Geometry check sheet. Reference: the model listing, model coordinates, mm. Face numbers are marked on the shaded views. Coordinates: 2 decimals unless noted, no trailing zeros. Write each loop counter-clockwise with the first axis right and the second up, starting at its lowest first coordinate (ties: lowest second). Pieces come first, ordered by that corner, then holes. Notation, with made-up numbers: (-34, 37) -> (-15, 37) arc R14 ccw to (-15, 51) -> close; hole circle Ø7 at (70, 18.25). An arc over 180 degrees is marked (long way). Answer as CSV lines item,"result".
```python
from build123d import *

# Parameters (mm, degrees)
SKETCH1_R           = 30.5
SKETCH1_R_2         = 17.5
BOSS_EXTRUDE1_DEPTH = 15
SKETCH2_R           = 2
CUT_EXTRUDE1_DEPTH  = 15
FILLET1_R           = 1
FILLET2_R           = 0.5


with BuildPart() as part:
    # Sketch1 → Boss-Extrude1 (new body)
    with BuildSketch(Plane(origin=(0, 0, 0), x_dir=(1, 0, 0), z_dir=(0, 1, 0))):
        with Locations(Location((0, 0, 0), (0, 0, 270))):
            Circle(SKETCH1_R)
        with Locations(Location((0, 0, 0), (0, 0, 270))):
            Circle(SKETCH1_R_2, mode=Mode.SUBTRACT)
    extrude(amount=BOSS_EXTRUDE1_DEPTH)

    # Sketch2 → Cut-Extrude1 (cut)
    with BuildSketch(Plane(origin=(0, 15, 0), x_dir=(1, 0, 0), z_dir=(0, 1, 0))):
        with Locations(Location((0, 22.5, 0), (0, 0, 270))):
            Circle(SKETCH2_R)
        with Locations(Location((15.909902577, 15.909902577, 0), (0, 0, 270))):
            Circle(SKETCH2_R)
        with Locations(Location((22.5, 0, 0), (0, 0, 270))):
            Circle(SKETCH2_R)
        with Locations(Location((15.909902577, -15.909902577, 0), (0, 0, 270))):
            Circle(SKETCH2_R)
        with Locations(Location((0, -22.5, 0), (0, 0, 270))):
            Circle(SKETCH2_R)
        with Locations(Location((-15.909902577, -15.909902577, 0), (0, 0, 270))):
            Circle(SKETCH2_R)
        with Locations(Location((-22.5, 0, 0), (0, 0, 270))):
            Circle(SKETCH2_R)
        with Locations(Location((-15.909902577, 15.909902577, 0), (0, 0, 270))):
            Circle(SKETCH2_R)
    extrude(amount=-CUT_EXTRUDE1_DEPTH, mode=Mode.SUBTRACT)

    # Fillet1
    fillet1_edges = [part.edges().sort_by_distance(p)[0] for p in [
        (0, 0, -17.5),
        (0, 15, -17.5),
    ]]
    fillet(fillet1_edges, radius=FILLET1_R)

    # Fillet2
    fillet2_edges = [part.edges().sort_by_distance(p)[0] for p in [
        (0, 0, -30.5),
        (0, 15, -30.5),
    ]]
    fillet(fillet2_edges, radius=FILLET2_R)


solid = part.part
```
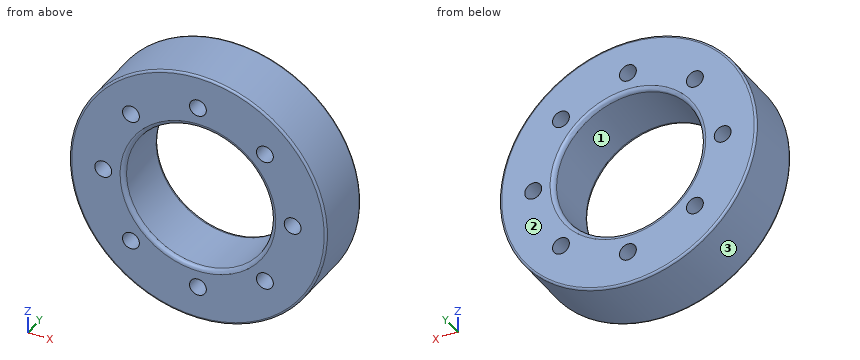
Item 1: Thickness scan on probe 1 along X at (y, z) = (10, 0); probe 2 along Z at (x, y) = (15.5, 10.5); probe 3 along Z at (x, y) = (23, 3.25). Record the ranges inside material, lowest first.
Responses:
probe 1,"x = -30.5 to -24.5, -20.5 to -17.5, 17.5 to 20.5, 24.5 to 30.5"
probe 2,"z = -26.27 to -17.87, -13.95 to -8.12, 8.12 to 13.95, 17.87 to 26.27"
probe 3,"z = -20.03 to -1.94, 1.94 to 20.03"
Item 2: Cross-section at A-A, the plane z = 0. Record the cut outline in (x, y).
Responses:
outline,"(-30.5, 0.5) arc R0.5 ccw to (-30, 0) -> (-24.5, 0) -> (-24.5, 15) -> (-30, 15) arc R0.5 ccw to (-30.5, 14.5) -> close; (-20.5, 0) -> (-18.5, 0) arc R1 ccw to (-17.5, 1) -> (-17.5, 14) arc R1 ccw to (-18.5, 15) -> (-20.5, 15) -> close; (17.5, 1) arc R1 ccw to (18.5, 0) -> (20.5, 0) -> (20.5, 15) -> (18.5, 15) arc R1 ccw to (17.5, 14) -> close; (24.5, 0) -> (30, 0) arc R0.5 ccw to (30.5, 0.5) -> (30.5, 14.5) arc R0.5 ccw to (30, 15) -> (24.5, 15) -> close"
Item 3: Depth check by flat-ended pin: pin 1 Ø4.5 at (x, z) = (15.91, 15.91) entering from +Y; pin 2 Ø5 at (y, z) = (9.5, 7) entering from -X; pin 3 Ø1.5 at (x, y) = (-16.5, 5.5) entering from +Z; pin 4 Ø1.5 at (x, y) = (-8, 6) entering from +Z. Enter the tip coordinate at first touch or a pass-through.
Responses:
pin 1,"stops at y = 15"
pin 2,"stops at x = -30.17"
pin 3,"stops at z = 26.12"
pin 4,"stops at z = 29.63"
Item 4: Cross-section at B-B, the plane y = 8. Count the separate pieces of the cut face and the enclosed holes in it, plus the area to 3 significant figures.
Responses:
separate pieces,"1"
enclosed holes,"9"
area,"1,860 mm2"
Item 5: Release check for a two-part mould opening along X. For the marked faces 1, 2 and 3 record: +X half, -X half, draft (parallel to the pull), parting line (faces both ways), or undercut.
Responses:
face 1,"undercut"
face 2,"draft"
face 3,"parting line"
